Autodesk Inventor part; units mm, degrees
ref_plane "Arbeitsebene1" through (0, 0, 5) normal (0, 0, 1) x (1, 0, 0)
ref_plane "Arbeitsebene2" through (0, 0, -5) normal (0, 0, 1) x (1, 0, 0)
ref_plane "Arbeitsebene3" through (0, 0, 0) normal (0, 1, 0) x (-1, 0, 0)
sketch "Skizze1" plane through (0, 0, 0) normal (1, 0, 0) x (0, 1, 0)
  circle A0 centre (0, 12.5) radius 6.5
  circle A1 centre (0, -12.5) radius 6.5
  line L0 (6.5, 12.5) -> (6.5, -12.5)
  line L1 (-6.5, -12.5) -> (-6.5, 12.5)
  point P0 (0, 0)
  dimension "d0" = 13
  dimension "d1" = 13
  dimension "d2" = 12.5
  dimension "d3" = 12.5
extrude "Extrusion1" add sketch "Skizze1" along normal blind 10
sketch "Skizze2" plane through (0, 0, 0) normal (-1, 0, 0) x (0, 0, 1)
  arc A0 (-12.5, 6.5) -> (-12.5, -6.5) centre (-12.5, 0) ccw
  circle A1 centre (-12.5, 0) radius 5.05
  arc A2 (12.5, -6.5) -> (12.5, 6.5) centre (12.5, 0) ccw
  circle A3 centre (12.5, 0) radius 5.05
  point P0 (0, 0)
  dimension "d8" = 10.1
  dimension "d9" = 10.1
extrude "Extrusion2" cut sketch "Skizze2" against normal blind 6
ref_plane "Arbeitsebene1" through (0, 0, 5) normal (0, 0, 1) x (1, 0, 0)
sketch "Skizze4" plane through (0, 0, 5) normal (0, 0, 1) x (1, 0, 0)
  line L0 (10, -6.5) -> (10, 6.5)
  line L1 (27.9456, 6.5) -> (10, 6.5)
  line L2 (27.9456, -6.5) -> (10, -6.5)
  line L3 (0, -6.5) -> (0, 6.5)
  line L4 (27.9456, 6.5) -> (34.4456, 6.5)
  line L5 (34.4456, 6.5) -> (34.4456, -6.5)
  line L6 (34.4456, -6.5) -> (27.9456, -6.5)
  point P0 (0, 0)
  point P1 (0, 0)
extrude "Extrusion3" add sketch "Skizze4" along normal blind 6
ref_plane "Arbeitsebene2" through (0, 0, -5) normal (0, 0, 1) x (1, 0, 0)
sketch "Skizze5" plane through (0, 0, -5) normal (0, 0, 1) x (1, 0, 0)
  line L0 (34.4456, 6.5) -> (10, 6.5)
  line L1 (10, 6.5) -> (10, -6.5)
  line L2 (27.9456, 6.5) -> (10, 6.5)
  line L3 (10, -6.5) -> (34.4456, -6.5)
  line L4 (27.9456, -6.5) -> (10, -6.5)
  line L5 (34.4456, -6.5) -> (34.4456, 6.5)
  line L6 (27.9456, 6.5) -> (34.4456, 6.5)
  line L7 (34.4456, 6.5) -> (34.4456, -6.5)
  line L8 (34.4456, -6.5) -> (27.9456, -6.5)
  point P0 (0, 0)
  point P1 (27.9456, 0)
  dimension "d26" = 24.4456
  dimension "d27" = 13
extrude "Extrusion4" add sketch "Skizze5" against normal blind 6
sketch "Skizze6" plane through (0, 0, -11) normal (0, 0, -1) x (-1, 0, 0)
  arc A0 (-27.9456, 6.5) -> (-27.9456, -6.5) centre (-27.9456, 0) ccw
  circle A1 centre (-27.9456, 0) radius 5.1
  point P0 (0, 0)
  dimension "d20" = 10.2
extrude "Extrusion5" cut sketch "Skizze6" against normal through all
ref_plane "Arbeitsebene3" through (0, 0, 0) normal (0, 1, 0) x (-1, 0, 0)
ref_plane "Arbeitsebene4" through (0, 0, 0) normal (0, 0, 1) x (1, 0, 0)
properties part number "ObenMotor"
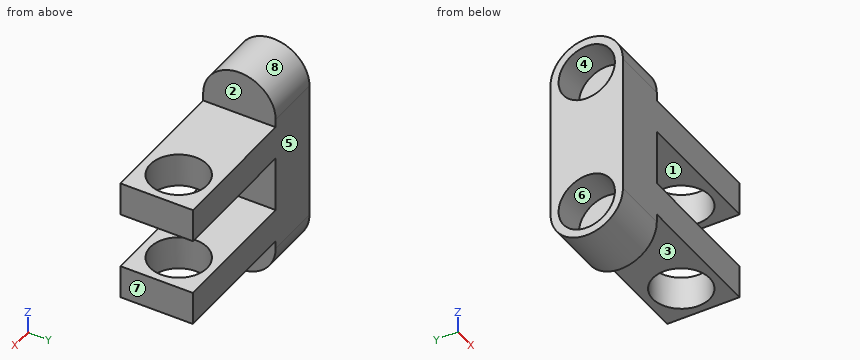
Verification items for the finished model (mm, model axes). Face numbers are marked on the shaded views. A direction names the side the tool comes from. Coordinates: 2 decimals unless noted, no trailing zeros. Loops run counter-clockwise (first coordinate to the right, second up) from the corner with the lowest first, then second, coordinate; pieces in that order, holes last. Notation, with made-up numbers: (-6, 18.5) -> (25, 18.5) arc R24 ccw to (25, 37.5) -> close; hole circle Ø10 at (63, 26). An arc over 180 degrees is marked (long way). Write each question's results on one line, items separated by ' | '.
Item 1: Section check A-A, the plane y = 0. Enter the section's corners in (x, z).
Found:
outline: (0, -19) -> (10, -19) -> (10, -11) -> (22.85, -11) -> (22.85, -5) -> (10, -5) -> (10, 5) -> (22.85, 5) -> (22.85, 11) -> (10, 11) -> (10, 19) -> (0, 19) -> (0, 17.55) -> (6, 17.55) -> (6, 7.45) -> (0, 7.45) -> (0, -7.45) -> (6, -7.45) -> (6, -17.55) -> (0, -17.55) -> close; (33.05, -11) -> (34.45, -11) -> (34.45, -5) -> (33.05, -5) -> close; (33.05, 5) -> (34.45, 5) -> (34.45, 11) -> (33.05, 11) -> close
Item 2: Section check B-B, the plane z = -6.5. Enter the section's corners in (x, y), plus the area to 3 significant figures.
Found:
outline: (0, -6.5) -> (34.45, -6.5) -> (34.45, 6.5) -> (0, 6.5) -> close; hole circle Ø10.2 at (27.95, 0) | area: 366 mm2
Item 3: Section check D-D, the plane z = 16.5. Enter the section's corners in (x, y).
Found:
outline: (0, -5.12) -> (10, -5.12) -> (10, 5.12) -> (0, 5.12) -> (0, 3.08) -> (6, 3.08) -> (6, -3.08) -> (0, -3.08) -> close
Item 4: Mould release check, pull along Y, two halves, no side actions. Record for the marked faces 6, 7 and 8: +Y half, -Y half, draft (parallel to the pull), parting line (faces both ways), or undercut.
Found:
face 6: undercut | face 7: draft | face 8: parting line
Item 5: Tool access check on the marked faces 1, 2, 3, 4 and 5. Record the directions out of +Z, -Z, +X, -X, +Y, -Y that give a thin tool (end or side, any length) a straight path to the whole face; none if there is none.
Found:
face 1: +X, +Y, -Y | face 2: +Z, +X, +Y, -Y | face 3: -Z, +X, +Y, -Y | face 4: -X | face 5: +Z, -Z, +X, -X, +Y
Item 6: Gauge pin test, flat ends, axial feed: pin 1 (6.5 mm diameter, centred on x = 21, y = -1, fed in from -Z); pin 2 (3 mm diameter, centred on y = 2, z = -11, fed in from -X); pin 3 (4 mm diameter, centred on y = 2, z = 7.5, fed in from -X); pin 4 (6.5 mm diameter, centred on y = 3, z = -15.5, fed in from +X). Record the tip position at first contact, or that the pin passes through.
Found:
pin 1: stops at z = -11 | pin 2: stops at x = 6 | pin 3: stops at x = 0 | pin 4: stops at x = 10
Item 7: Section check C-C, the plane x = 8. Enter the section's corners in (y, z), plus the area to 3 significant figures.
Found:
outline: (-6.5, -12.5) arc R6.5 ccw to (6.5, -12.5) -> (6.5, 12.5) arc R6.5 ccw to (-6.5, 12.5) -> close | area: 458 mm2
Item 8: Material ranges on L1, parallel to Z at x = 18, y = 2.5; L2, parallel to Y at x = 3.9, z = -12.5; L3, parallel to X at y = 0.25, z = -7.5, recorded low to high.
Found:
L1: z = -11 to -5, 5 to 11 | L2: y = -6.5 to -5.05, 5.05 to 6.5 | L3: x = 6 to 22.85, 33.04 to 34.45
